```python
from build123d import *

# Parameters (mm, degrees)
F1_DEPTH = 30
F2_DEPTH = 20


with BuildPart() as f1:
    # F0 (on Front) → F1 (new body)
    with BuildSketch(Plane.XZ):
        with BuildLine():
            Line((0, -30), (0, 0))
            Line((0, 0), (30, 30))
            Line((30, 30), (50, 30))
            ThreePointArc((50, 30), (57.071068, 32.928932), (60, 40))
            Line((60, 40), (60, 50))
            ThreePointArc((60, 50), (57.071068, 57.071068), (50, 60))
            Line((50, 60), (-40, 60))
            ThreePointArc((-40, 60), (-47.071068, 57.071068), (-50, 50))
            Line((-50, 50), (-50, -30))
            ThreePointArc((-50, -30), (-47.071068, -37.071068), (-40, -40))
            Line((-40, -40), (-10, -40))
            ThreePointArc((-10, -40), (-2.928932, -37.071068), (0, -30))
        make_face()
        Polygon((-45, -35), (-45, 15), (-45, 55), (-5, 55), (-5, -35), align=None, mode=Mode.SUBTRACT)
        Polygon((-45, 55), (-45, 15), (-45, -35), (-5, -35), (-5, 55), align=None)
    extrude(amount=-F1_DEPTH)

    # F0 (on Front) → F2 (cut)
    with BuildSketch(Plane.XZ):
        Polygon((-45, 55), (-45, 15), (-45, -35), (-5, -35), (-5, 55), align=None)
    extrude(amount=-F2_DEPTH, mode=Mode.SUBTRACT)


solid = f1.part
```
Design review of the part built by this model. Coordinates are the model's own, in mm. A direction names the side the tool comes from. Give positions to 0.01 mm unless a question says otherwise; leave off trailing zeros. Order: outer loops, then holes, each group sorted by start corner. A loop starts at its lowest first (then second) coordinate and runs counter-clockwise, first axis right, second up. Notation, with made-up numbers: M 27,53.25 L 45,53.25 A17 cw 45,62.25 Z; hole C -3,-24 d7. An arc over 180 degrees is marked long. One line per question, with ' | ' between items. Start each with the question number.
Q1. We need section A-A (y = 6.25). Write out the cut boundary in (x, z), plus the area to 3 significant figures.
Q2. We need section C-C (y = 26.25). Write out the cut boundary in (x, z), plus the area to 3 significant figures.
Q3. We need section D-D (x = -12). Write out the cut boundary in (y, z).
Q4. The part is to be moulded in two halves that separate along Y. For faces 4 (the face through (-8, 30, 22)), 5 (the face through (-25, 20, 11)), 6 (the face through (-47.15, 14.79, -36.99)), say which applies: +Y half, -Y half, draft (parallel to the pull), parting line (faces both ways), or undercut.
Q5. We need section B-B (z = -22.5). Write out the cut boundary in (x, y).
Q6. For pin 1 Ø15 at (y, z) = (9.5, -9) entering from +X; pin 2 Ø10 at (y, z) = (8, 31.5) entering from +X; pin 3 Ø10 at (x, y) = (42, 22.5) entering from -Z, all flat-tipped, find the tip position at first contact; note any pin that passes through.
Q7. Machinability: for faces 1 (the face through (-25, 10, -35)), 2 (the face through (60, 15, 45)), 3 (the face through (40, 15, 30)), which of the approach directions +Z, -Z, +X, -X, +Y, -Y give a long, thin tool a straight path to every point of the face, cutting with its end or side? Answer none if there is none.
Q8. For L1, parallel to X at y = 1.75, z = -9.5; L2, parallel to Z at x = -23, y = 10.5; L3, parallel to Y at x = -28, z = -18, list the stretches that pass through material, from the lowest coordinate up. Write a range as [from, to].
Returned:
1) outline: M -50,-30 A10 ccw -40,-40 L -10,-40 A10 ccw 0,-30 L 0,0 L 30,30 L 50,30 A10 ccw 60,40 L 60,50 A10 ccw 50,60 L -40,60 A10 ccw -50,50 Z; hole M -45,-35 L -5,-35 L -5,55 L -45,55 Z | area: 3,540 mm2
2) outline: M -50,-30 A10 ccw -40,-40 L -10,-40 A10 ccw 0,-30 L 0,0 L 30,30 L 50,30 A10 ccw 60,40 L 60,50 A10 ccw 50,60 L -40,60 A10 ccw -50,50 Z | area: 7,140 mm2
3) outline: M 0,-40 L 30,-40 L 30,60 L 0,60 L 0,55 L 20,55 L 20,-35 L 0,-35 Z
4) face 4: +Y half | face 5: -Y half | face 6: draft
5) outline: M -50,0 L -45,0 L -45,20 L -5,20 L -5,0 L 0,0 L 0,30 L -50,30 Z
6) pin 1: x = 0 | pin 2: x = 59.37 | pin 3: z = 30
7) face 1: -Y | face 2: +Z, -Z, +X, +Y, -Y | face 3: -Z, +X, +Y, -Y
8) L1: [-50, -45], [-5, 0] | L2: [-40, -35], [55, 60] | L3: [20, 30]
